The model under review builds one solid part; all positions refer to its coordinate system, in mm. A direction names the side the tool comes from. Round coordinates to 2 decimals unless told otherwise and drop trailing zeros. Order: outer loops, then holes, each group sorted by start corner. A loop starts at its lowest first (then second) coordinate and runs counter-clockwise, first axis right, second up. Notation, with made-up numbers: M -36.75,-22.75 L 12.25,-22.75 A24 cw 12.25,12.25 Z; hole C 59,-15.5 d3. An arc over 180 degrees is marked long. Use a Markdown table: item, result. Add a question column.
1. For faces 4 (the flat face through (4, 18.5, 0)), 5 (the flat face through (4, 17.5, 0)), list the 3-axis set-ups (+Z, -Z, +X, -X, +Y, -Y) from which the entire face can be reached by the end or side of a thin tool; tool diameter is ignored.
2. Consider section D-D on y = 11.75. State the section outline as (x, z) points, then the cut area to 3 significant figures.
3. Consider section C-C on y = 5. State the section outline as (x, z) points.
4. Insertion check: P1, Ø2, axis at y = 13, z = -10.5, coming from the +X side; P2, Ø2, axis at x = -17, z = -22.5, coming from the +Y side; P3, Ø8, axis at y = 7.5, z = 0, coming from the +X side. Each pin has a flat end and moves straight along its axis. Give the tip position at first contact, or say it passes through.
5. Consider section B-B on z = 0. State the section outline as (x, y) points.
6. Consider section A-A on x = 0. State the section outline as (y, z) points, then the cut area to 3 significant figures.
7. To check wall thickness, follow probe 1 along X at (y, z) = (2.25, 0); probe 2 along Y at (x, z) = (16.5, -3); probe 3 along Z at (x, y) = (4.5, 7.5). State the ranges of each line that lie inside material, in increasing order.
8. The part is to be moulded in two halves that separate along X. For faces 1 (the cylindrical face through (11.107, 4.19, -26.789)), 2 (the cylindrical face through (-1.612, 18.007, -2.103)), 3 (the flat face through (-24, 0, 15)), say which applies: +X half, -X half, draft (parallel to the pull), parting line (faces both ways), or undercut.
from build123d import *

# Parameters (mm, degrees)
SKETCH2_R          = 2.65
CUT_EXTRUDE1_DEPTH = 45.991665959


with BuildPart() as part:
    # Sketch1 → Revolve-Thin1 (revolve)
    with BuildSketch(Plane.XY, mode=Mode.PRIVATE) as revolve_thin1_sk:
        with BuildLine():
            Line((0, 18.5), (-19, 18.5))
            ThreePointArc((-19, 18.5), (-26.071067812, 15.571067812), (-29, 8.5))
            Line((-29, 8.5), (-29, 0))
            Line((-29, 0), (-28, 0))
            Line((-28, 0), (-28, 8.5))
            ThreePointArc((-28, 8.5), (-25.363961031, 14.863961031), (-19, 17.5))
            Line((-19, 17.5), (0, 17.5))
            Line((0, 17.5), (0, 18.5))
        make_face()
    revolve(revolve_thin1_sk.sketch.rotate(Axis((0, 0, 0), (0, 1, 0)), 270), axis=Axis((0, 0, 0), (0, 1, 0)))

    # Sketch2 → Cut-Extrude1 (cut, through all)
    with BuildSketch(Plane(origin=(0, 18.5, 0), x_dir=(1, 0, 0), z_dir=(0, 1, 0))):
        with Locations(Location((0, 0, 0), (0, 0, 270))):
            Circle(SKETCH2_R)
    extrude(amount=-CUT_EXTRUDE1_DEPTH, mode=Mode.SUBTRACT)


solid = part.part
Answer block:
| question | item | result |
|---|---|---|
| 1 | face 4 | +Z, -Z, +X, -X, +Y |
| 1 | face 5 | -Y |
| 2 | outline | C 0,0 d56.91; hole C 0,0 d54.79 |
| 2 | area | 187 mm^2 |
| 3 | outline | C 0,0 d58; hole C 0,0 d56 |
| 4 | P1 | x = 26.5 |
| 4 | P2 | y = 14.22 |
| 4 | P3 | x = 29 |
| 5 | outline | M -29,0 L -28,0 L -28,8.5 A9 cw -19,17.5 L -2.65,17.5 L -2.65,18.5 L -19,18.5 A10 ccw -29,8.5 Z; M 2.65,17.5 L 19,17.5 A9 cw 28,8.5 L 28,0 L 29,0 L 29,8.5 A10 ccw 19,18.5 L 2.65,18.5 Z |
| 6 | outline | M 0,-29 L 8.5,-29 A10 ccw 18.5,-19 L 18.5,-2.65 L 17.5,-2.65 L 17.5,-19 A9 cw 8.5,-28 L 0,-28 Z; M 0,28 L 8.5,28 A9 cw 17.5,19 L 17.5,2.65 L 18.5,2.65 L 18.5,19 A10 ccw 8.5,29 L 0,29 Z |
| 6 | area | 79.5 mm^2 |
| 7 | probe 1 | -29 to -28, 28 to 29 |
| 7 | probe 2 | 17.5 to 18.5 |
| 7 | probe 3 | -28.65 to -27.64, 27.64 to 28.65 |
| 8 | face 1 | parting line |
| 8 | face 2 | undercut |
| 8 | face 3 | draft |
